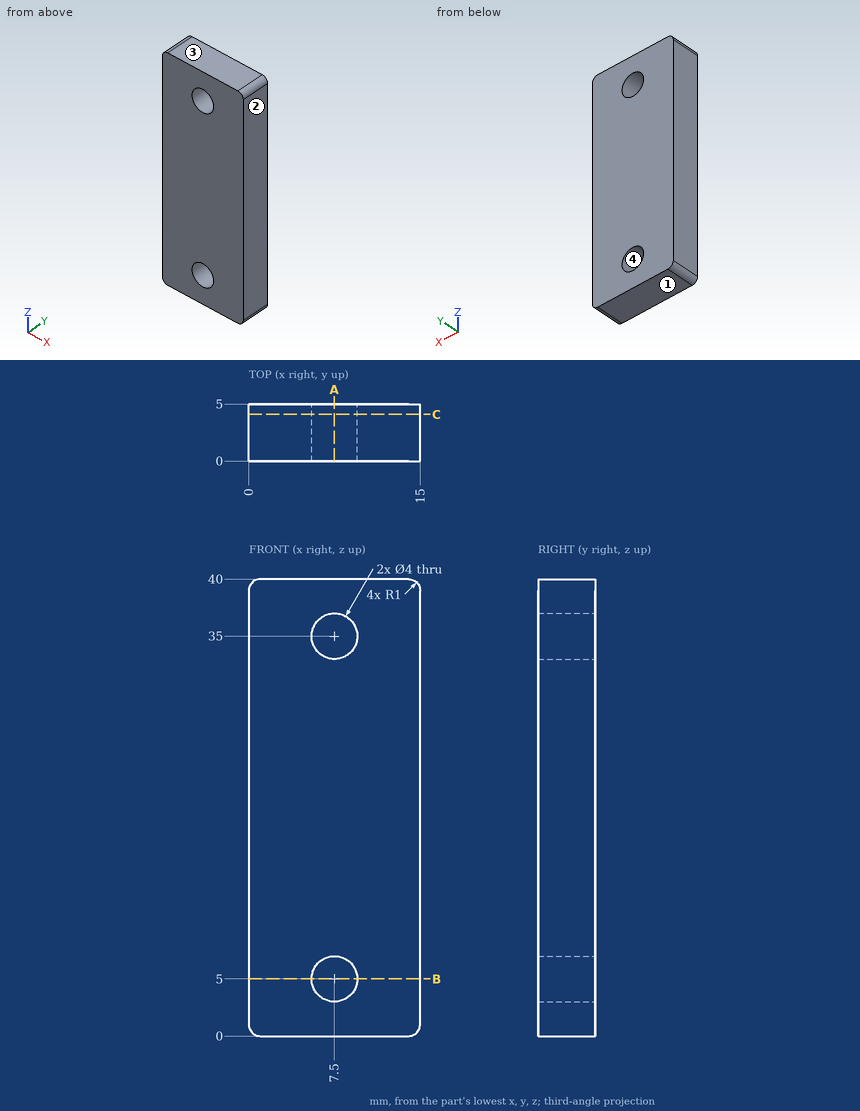
Print and shaded views of the part. All mm, measured from the part's lowest x, y and z. Round coordinates to 2 decimals unless told otherwise and drop trailing zeros. Write each loop counter-clockwise with the first axis right and the second up, starting at its lowest first coordinate (ties: lowest second). Pieces come first, ordered by that corner, then holes. Notation, with made-up numbers: (51, 14.25) -> (78, 14.25) arc R14 cw to (78, 28.25) -> close; hole circle Ø8 at (4.5, 61). An arc over 180 degrees is marked (long way). Return JSON: item names as keys, results as strings. Group by question number.
Q1. Probe L1, parallel to Z at x = 7.5, y = 1.2; L2, parallel to X at y = 3.75, z = 35; L3, parallel to Z at x = 7, y = 4.75. List the from-to ranges inside material, lowest first. Write a range as [from, to].
Q2. Saw through at B-B on z = 5. Write the cut outline in (x, y), plus the area to 3 significant figures.
Q3. Saw through at C-C on y = 4.1. Write the cut outline in (x, z).
Q4. Mould opens along Z. For the marked faces 1, 2, 3 and 4 say: pulls with the +Z half, pulls with the -Z half, needs draft (parallel to the pull), parting line crosses it, or undercut.
Q5. Saw through at A-A on x = 7.5. Write the cut outline in (y, z).
Q6. Pin check, flat tip, straight feed: pin 1 (3 mm diameter, centred on x = 7.5, z = 35, fed in from -Y). Stop position of the tip, or through.
Answer:
{
 "1": {"L1": "[0, 3], [7, 33], [37, 40]", "L2": "[0, 5.5], [9.5, 15]", "L3": "[0, 3.06], [6.94, 33.06], [36.94, 40]"},
 "2": {"outline": "(0, 0) -> (5.5, 0) -> (5.5, 5) -> (0, 5) -> close; (9.5, 0) -> (15, 0) -> (15, 5) -> (9.5, 5) -> close", "area": "55.0 mm2"},
 "3": {"outline": "(0, 1) arc R1 ccw to (1, 0) -> (14, 0) arc R1 ccw to (15, 1) -> (15, 39) arc R1 ccw to (14, 40) -> (1, 40) arc R1 ccw to (0, 39) -> close; hole circle Ø4 at (7.5, 5); hole circle Ø4 at (7.5, 35)"},
 "4": {"face 1": "pulls with the -Z half", "face 2": "needs draft", "face 3": "pulls with the +Z half", "face 4": "undercut"},
 "5": {"outline": "(0, 0) -> (5, 0) -> (5, 3) -> (0, 3) -> close; (0, 7) -> (5, 7) -> (5, 33) -> (0, 33) -> close; (0, 37) -> (5, 37) -> (5, 40) -> (0, 40) -> close"},
 "6": {"pin 1": "through"}
}
